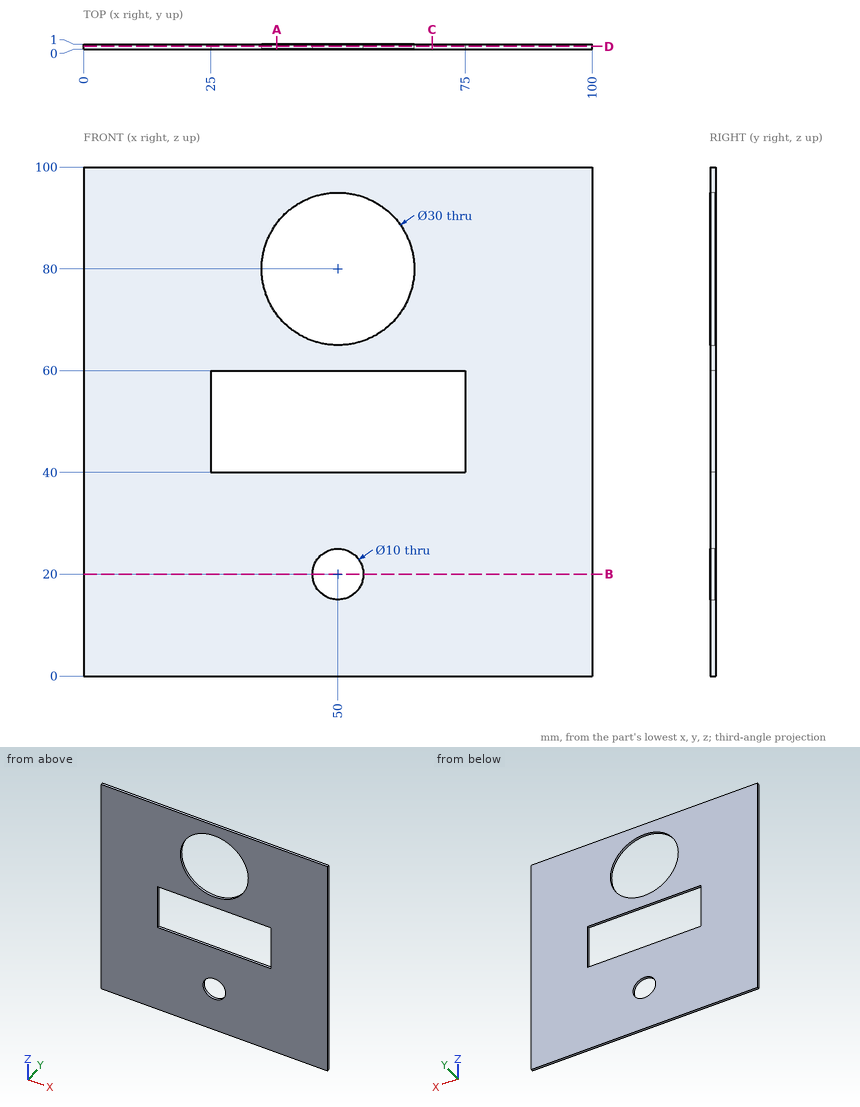
Answer from the drawing. Dimensions are ordinates in mm from the lowest x, y and z of the part. Round coordinates to 2 decimals unless told otherwise and drop trailing zeros. Loops run counter-clockwise (first coordinate to the right, second up) from the corner with the lowest first, then second, coordinate; pieces in that order, holes last.
1) Given P1, Ø8, axis at x = 50, z = 20, coming from the -Y side, flat-ended and moving along its own axis, determine where the tip first touches the part or whether it passes through.
Outcome:
P1: passes through
2) Consider line 1 (X direction, y = 0.6, z = 20); line 2 (X direction, y = 0.5, z = 80); line 3 (Z direction, x = 50.5, y = 0.6). Determine where each line is inside the solid, lowest interval first.
Outcome:
line 1: x = 0 to 45, 55 to 100
line 2: x = 0 to 35, 65 to 100
line 3: z = 0 to 15.03, 24.97 to 40, 60 to 65.01, 94.99 to 100
3) A cutting plane is placed at B-B on z = 20. Determine the outline of the cut face in (x, y), plus the area to 3 significant figures.
Outcome:
outline: (0, 0) - (45, 0) - (45, 1) - (0, 1) - close; (55, 0) - (100, 0) - (100, 1) - (55, 1) - close
area: 90.0 mm2
4) A cutting plane is placed at C-C on x = 68.5. Determine the outline of the cut face in (y, z).
Outcome:
outline: (0, 0) - (1, 0) - (1, 40) - (0, 40) - close; (0, 60) - (1, 60) - (1, 100) - (0, 100) - close
5) A cutting plane is placed at A-A on x = 38. Determine the outline of the cut face in (y, z), plus the area to 3 significant figures.
Outcome:
outline: (0, 0) - (1, 0) - (1, 40) - (0, 40) - close; (0, 60) - (1, 60) - (1, 71) - (0, 71) - close; (0, 89) - (1, 89) - (1, 100) - (0, 100) - close
area: 62.0 mm2
6) A cutting plane is placed at D-D on y = 0.55. Determine the outline of the cut face in (x, z).
Outcome:
outline: (0, 0) - (100, 0) - (100, 100) - (0, 100) - close; hole (25, 40) - (75, 40) - (75, 60) - (25, 60) - close; hole circle Ø30 at (50, 80); hole circle Ø10 at (50, 20)
